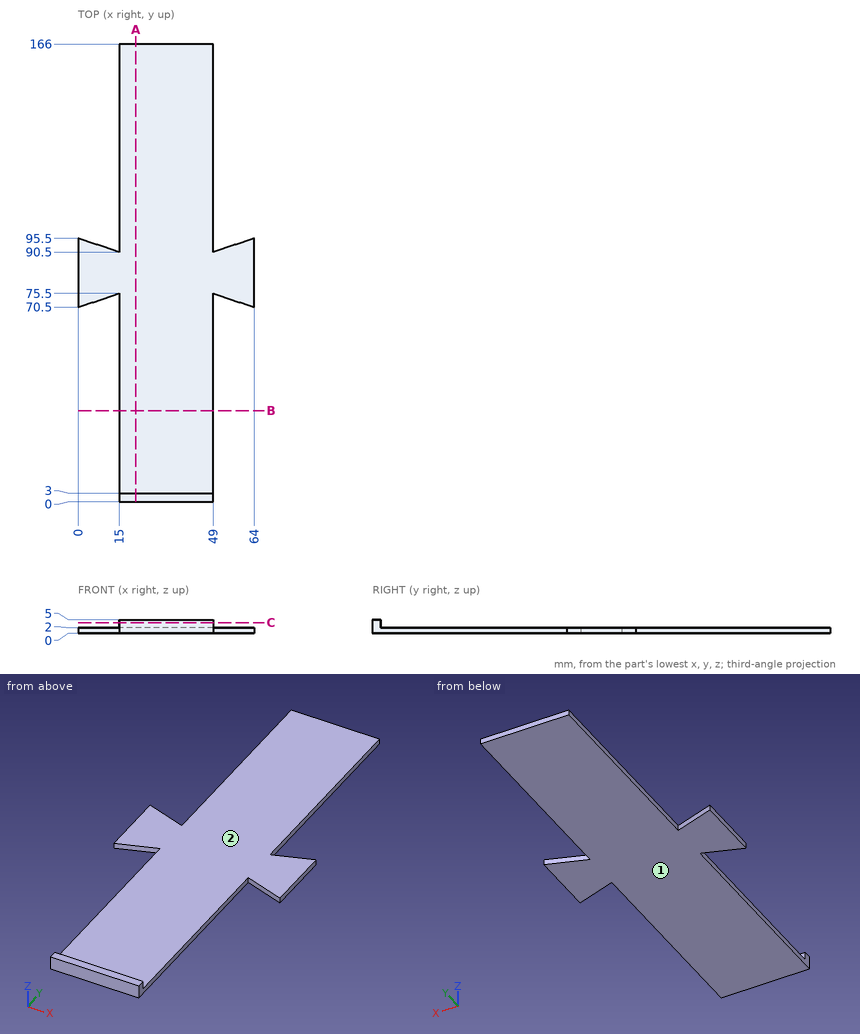
The drawing under review shows one solid part. Ordinate dimensions are in mm from its lowest x, y, z. A direction names the side the tool comes from. Coordinates: 2 decimals unless noted, no trailing zeros. Order: outer loops, then holes, each group sorted by start corner. A loop starts at its lowest first (then second) coordinate and runs counter-clockwise, first axis right, second up. Notation, with made-up numbers: (68, 51) - (114, 51) arc R38 cw to (114, 89) - close; hole circle Ø7 at (78.5, 68.5). An arc over 180 degrees is marked (long way). Put each result on its own line as item: value.
1) Take a section at C-C, the plane z = 3.9. Give the boundary of the cut face in (x, y), and give its area (3 significant figures).
Response values:
outline: (15, 0) - (49, 0) - (49, 3) - (15, 3) - close
area: 102 mm²
2) Insertion check: P1, Ø2.5, axis at y = 30.5, z = 2.5, coming from the -X side; P2, Ø0.9, axis at x = 34.5, z = 3, coming from the +Y side; P3, Ø1.6, axis at y = 116, z = 1, coming from the +X side. Each pin has a flat end and moves straight along its axis. Give the tip position at first contact, or say it passes through.
Response values:
P1: stops at x = 15
P2: stops at y = 3
P3: stops at x = 49
3) Tool access review of the marked faces 1 and 2: name each direction out of +Z, -Z, +X, -X, +Y, -Y from which nothing blocks a thin tool from reaching the whole face with its end or side.
Response values:
face 1: -Z, +X, -X, +Y, -Y
face 2: +Z, +X, -X, +Y
4) Wall thickness on L1, parallel to Z at x = 35.5, y = 70.5; L2, parallel to Y at x = 29, z = 3.45; L3, parallel to X at y = 60.5, z = 0.6: over which ranges is each line inside the solid? List them lowest first. Write a range as from..to.
Response values:
L1: z = 0..2
L2: y = 0..3
L3: x = 15..49
5) Take a section at A-A, the plane x = 21. Give the boundary of the cut face in (y, z), and give its area (3 significant figures).
Response values:
outline: (0, 0) - (166, 0) - (166, 2) - (3, 2) - (3, 5) - (0, 5) - close
area: 341 mm²
6) Take a section at B-B, the plane y = 33. Give the boundary of the cut face in (x, z), and give its area (3 significant figures).
Response values:
outline: (15, 0) - (49, 0) - (49, 2) - (15, 2) - close
area: 68.0 mm²
